from build123d import *

# Parameters (mm, degrees)
SKETCH001_R     = 22.5
SKETCH001_R_2   = 8
SKETCH001_R_3   = 1.25
SKETCH001_R_4   = 12
PAD_DEPTH       = 11
CHAMFER_SIZE    = 1
CHAMFER001_SIZE = 1
FILLET_R        = 1
FILLET001_R     = 1
CHAMFER002_SIZE = 0.5
CHAMFER003_SIZE = 0.2
CHAMFER004_SIZE = 0.2


with BuildPart() as part:
    # Sketch001 → Pad (new body)
    with BuildSketch(Plane.XY):
        with BuildLine():
            ThreePointArc((176.426018, 287.799835), (161.667114, 300.121263), (146.90821, 287.799835))
            Line((134.609123, 220.031978), (146.90821, 287.799835))
            ThreePointArc((134.609123, 220.031978), (161.667114, 187.621263), (188.725105, 220.031978))
            Line((176.426018, 287.799835), (188.725105, 220.031978))
        make_face()
        with Locations((161.667114, 215.121263)):
            Circle(SKETCH001_R, mode=Mode.SUBTRACT)
        with Locations((161.667114, 285.121263)):
            Circle(SKETCH001_R_2, mode=Mode.SUBTRACT)
        with Locations((171.626406, 290.871263)):
            Circle(SKETCH001_R_3, mode=Mode.SUBTRACT)
        with Locations((161.667114, 273.621263)):
            Circle(SKETCH001_R_3, mode=Mode.SUBTRACT)
        with Locations((151.707822, 290.871263)):
            Circle(SKETCH001_R_3, mode=Mode.SUBTRACT)
        with Locations((161.667114, 240.121263)):
            Circle(SKETCH001_R_3, mode=Mode.SUBTRACT)
        with Locations((186.667114, 215.121263)):
            Circle(SKETCH001_R_3, mode=Mode.SUBTRACT)
        with Locations((161.667114, 190.121263)):
            Circle(SKETCH001_R_3, mode=Mode.SUBTRACT)
        with Locations((136.667114, 215.121263)):
            Circle(SKETCH001_R_3, mode=Mode.SUBTRACT)
        with Locations((161.667114, 257.121263)):
            Circle(SKETCH001_R_4, mode=Mode.SUBTRACT)
    extrude(amount=PAD_DEPTH)

    # Chamfer
    chamfer_edges = [part.edges().sort_by_distance(p)[0] for p in [
        (139.167114, 215.121263, 11),
        (149.667114, 257.121263, 11),
    ]]
    chamfer(chamfer_edges, length=CHAMFER_SIZE)

    # Chamfer001
    chamfer001_edges = [part.edges().sort_by_distance(p)[0] for p in [
        (153.667114, 285.121263, 11),
    ]]
    chamfer(chamfer001_edges, length=CHAMFER001_SIZE)

    # Fillet
    fillet_edges = [part.edges().sort_by_distance(p)[0] for p in [
        (140.758666, 253.915906, 11),
        (161.667114, 300.121263, 11),
        (182.575562, 253.915906, 11),
        (161.667114, 187.621263, 11),
    ]]
    fillet(fillet_edges, radius=FILLET_R)

    # Fillet001
    fillet001_edges = [part.edges().sort_by_distance(p)[0] for p in [
        (140.758666, 253.915906, 0),
        (161.667114, 300.121263, 0),
        (182.575562, 253.915906, 0),
        (161.667114, 187.621263, 0),
    ]]
    fillet(fillet001_edges, radius=FILLET001_R)

    # Chamfer002
    chamfer002_edges = [part.edges().sort_by_distance(p)[0] for p in [
        (170.376406, 290.871263, 11),
        (160.417114, 273.621263, 11),
        (150.457822, 290.871263, 11),
    ]]
    chamfer(chamfer002_edges, length=CHAMFER002_SIZE)

    # Chamfer003
    chamfer003_edges = [part.edges().sort_by_distance(p)[0] for p in [
        (160.417114, 240.121263, 11),
    ]]
    chamfer(chamfer003_edges, length=CHAMFER003_SIZE)

    # Chamfer004
    chamfer004_edges = [part.edges().sort_by_distance(p)[0] for p in [
        (185.417114, 215.121263, 11),
        (160.417114, 190.121263, 11),
        (135.417114, 215.121263, 11),
    ]]
    chamfer(chamfer004_edges, length=CHAMFER004_SIZE)


solid = part.part
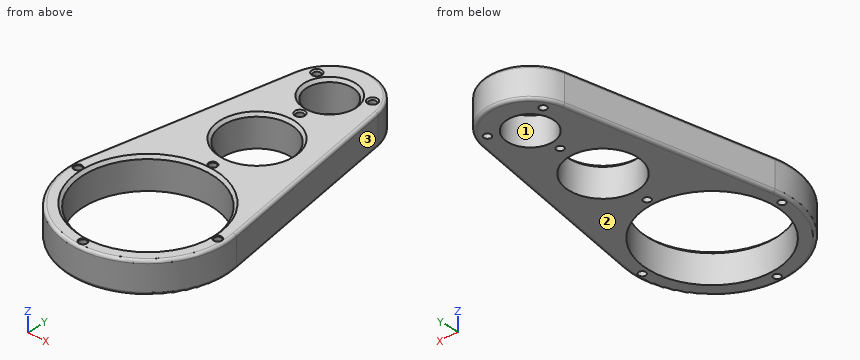
The model under review builds one solid part; all positions refer to its coordinate system, in mm. Face numbers are marked on the shaded views. Round coordinates to 2 decimals unless told otherwise and drop trailing zeros. Answer as CSV lines item,"result". Start each with the question number.
Q1. Clearance check with flat-ended pins moving along their axes: P1, Ø5, axis at x = 148, z = 4.5, coming from the -Y side; P2, Ø4, axis at x = 161.67, y = 240.12, coming from the +Z side; P3, Ø5, axis at x = 141, z = 9.5, coming from the -Y side; P4, Ø3, axis at x = 161.67, y = 273.62, coming from the +Z side. State where each tip first meets the part, or that it passes through.
Q2. Wall thickness on line 1 along Y through (x, z) = (170.5, 8); line 2 along Y through (x, z) = (159.5, 7.75); line 3 along Y through (x, z) = (153, 3.5): over which ranges is each line inside the solid? List them lowest first.
Q3. Consider section A-A, the plane z = 7. State how many separate pieces and enclosed holes the cut face has, then the cut area to 3 significant figures.
Q4. The part is to be moulded in two halves that separate along Y. For the marked faces 1, 2 and 3, say which applies: +Y half, -Y half, draft (parallel to the pull), parting line (faces both ways), or undercut.
Result set:
1,P1,"stops at y = 189.99"
1,P2,"stops at z = 11"
1,P3,"stops at y = 194.48"
1,P4,"stops at z = 10.75"
2,line 1,"y = 189.08 to 194.43, 235.81 to 249, 265.24 to 290.33, 291.41 to 297.24"
2,line 2,"y = 187.71 to 192.73, 237.52 to 245.32, 268.92 to 277.42, 292.82 to 299.96"
2,line 3,"y = 189.02 to 194.36, 235.88 to 248.82, 265.42 to 297.36"
3,separate pieces,"1"
3,enclosed holes,"10"
3,area,"2,290 mm²"
4,face 1,"undercut"
4,face 2,"draft"
4,face 3,"+Y half"
